Source: CAD feature listing. Evaluate the final solid. Frame: model axes, mm. A direction names the side the tool comes from. Coordinates: 2 decimals unless noted, no trailing zeros. Write each loop counter-clockwise with the first axis right and the second up, starting at its lowest first coordinate (ties: lowest second). Pieces come first, ordered by that corner, then holes. Notation, with made-up numbers: (-29, -36) -> (17, -36) arc R24 ccw to (17, -25) -> close; hole circle Ø3 at (41, 9.5). An arc over 180 degrees is marked (long way). One line per item, written item: value. Start each with the question number.
1. Section query B-B, the plane x = 214.25. Output: boundary loops of the cut face in (y, z).
2. Line query: line 1 (Y direction, x = 226.25, z = -12.25); line 2 (Y direction, x = 217.25, z = -2.25); line 3 (X direction, y = -2.25, z = -8.75). Output: solid intervals per line, ascending.
3. Section query C-C, the plane x = 227. Output: boundary loops of the cut face in (y, z), and give its area (3 significant figures).
4. First-contact query: P1, Ø4.5, axis at x = 224.5, z = -11.5, coming from the +Y side; P2, Ø4, axis at x = 214, y = -7, coming from the -Z side; P3, Ø6, axis at x = 212.5, y = -8.5, coming from the +Z side. Flat tips, straight axial feed; report the tip coordinate or a pass-through.
5. Section query D-D, the plane y = -1. Output: boundary loops of the cut face in (x, z).
6. Access query for faces 1 (the flat face through (228, -1, -9.9)), 2 (the flat face through (210.8, -11.8, -11.5)), 3 (the flat face through (228, -1, -1.2)). Directions: +Z, -Z, +X, -X, +Y, -Y. A direction counts if a zero-diameter tool reaches every point of the face in a straight line with its end or side. Return the directions, or none.
7. Section query A-A, the plane z = -13. Output: boundary loops of the cut face in (x, y).
Autodesk Inventor part; units mm, degrees
ref_plane "РабПлоскость1" through (116.75, -2.8, -7.7) normal (0, -1, 0) x (1, 0, 0)
ref_plane "YZ Plane" through (0, 0, 0) normal (1, 0, 0) x (0, 1, 0)
ref_plane "XZ Plane" through (0, 0, 0) normal (0, 1, 0) x (-1, 0, 0)
ref_plane "РабПлоскость1" through (116.75, -2.8, -7.7) normal (0, -1, 0) x (1, 0, 0)
sketch "Эскиз1" plane through (116.75, -2.8, -7.7) normal (0, -1, 0) x (1, 0, 0)
  line L0 (97, 9) -> (112.5, 9)
  line L1 (112.5, 9) -> (112.5, -9)
  line L2 (112.5, -9) -> (97, -9)
  line L3 (112.5, 2.2) -> (109.5, 2.2)
  line L4 (109.5, 2.2) -> (109.5, -6.5)
  line L5 (112.5, -6.5) -> (112.5, 2.2)
  line L6 (109.5, -6.5) -> (112.5, -6.5)
  line L7 (97, 9) -> (97, -9)
  point P0 (-116.75, 7.7)
  dimension "d9" = 15.5
  dimension "d10" = 3
  dimension "d11" = 8.7
  dimension "d13" = 2.5
extrude "Выдавливание1" add sketch "Эскиз1" along normal blind 1.5
sketch "Эскиз5" plane through (116.75, -2.8, -7.7) normal (0, 1, 0) x (1, 0, 0)
  line L0 (112.5, 9) -> (112.5, -9)
  line L1 (112.5, 2.2) -> (109.5, 2.2)
  line L2 (109.5, 2.2) -> (109.5, -6.5)
  line L3 (109.5, -6.5) -> (112.5, -6.5)
  line L4 (112.5, -6.5) -> (112.5, 2.2)
  line L5 (112.5, -9) -> (97, -9)
  point P0 (-116.75, -7.7)
  point P1 (112.5, -6.5)
  dimension "d14" = 3
  dimension "d15" = 8.7
  dimension "d16" = 2.5
extrude "Выдавливание5" add sketch "Эскиз5" along normal blind 2.8
sketch "Эскиз6" plane through (116.75, -4.3, -7.7) normal (0, -1, 0) x (1, 0, 0)
  line L0 (112.5, 9) -> (97, 9)
  line L1 (105.5, 9) -> (112.5, 9)
  line L2 (112.5, 9) -> (112.5, -9)
  line L3 (112.5, -9) -> (105.5, -9)
  line L4 (105.5, -9) -> (105.5, 9)
  point P0 (112.5, 9)
  dimension "d19" = 7
extrude "Выдавливание6" add sketch "Эскиз6" along normal blind 2.3
sketch "Эскиз7" plane through (116.75, -4.3, -7.7) normal (0, -1, 0) x (1, 0, 0)
  line L0 (97, 5.9073) -> (101.8, 5.9073)
  line L1 (101.8, 5.9073) -> (101.8, -5.6927)
  line L2 (101.8, -5.6927) -> (97, -5.6927)
  line L3 (97, -5.6927) -> (97, 5.9073)
  line L4 (97, 5.9073) -> (101.8, -5.6927) construction
  line L5 (101.8, 5.9073) -> (97, -5.6927) construction
  line L6 (97, 9) -> (97, -9)
  point P0 (99.4, 0.1073)
  point P1 (97, 0)
  dimension "d22" = 4.8
  dimension "d23" = 11.6
extrude "Выдавливание7" add sketch "Эскиз7" along normal blind 3.3
ref_plane "РабПлоскость3" through (116.75, -9.1, -7.7) normal (0, -1, 0) x (1, 0, 0)
sketch "Эскиз8" plane through (116.75, -9.1, -7.7) normal (0, -1, 0) x (1, 0, 0)
  line L0 (99.5911, -4.348) -> (90.6911, -4.348)
  line L1 (90.6911, -4.348) -> (90.6911, 4.252)
  line L2 (90.6911, 4.252) -> (99.5911, 4.252)
  line L3 (99.5911, 4.252) -> (99.5911, -4.348)
  line L4 (99.5911, -4.348) -> (90.6911, 4.252) construction
  line L5 (90.6911, -4.348) -> (99.5911, 4.252) construction
  point P0 (95.1411, -0.048)
  dimension "d27" = 8.9
  dimension "d28" = 8.6
extrude "Выдавливание8" add sketch "Эскиз8" along normal blind 2.7
sketch "Эскиз9" plane through (116.75, -11.8, -7.7) normal (0, -1, 0) x (1, 0, 0)
  line L0 (99.5911, 4.252) -> (90.6911, 4.252)
  line L1 (90.6911, 4.252) -> (90.6911, -4.348)
  line L2 (90.6911, -4.348) -> (99.5911, -4.348)
  line L3 (99.5911, -4.348) -> (99.5911, 4.252)
  circle A0 centre (95.1411, -0.048) radius 3.75
  line L4 (99.5911, -4.348) -> (99.5911, 4.252)
  line L5 (99.5911, -4.348) -> (90.6911, 4.252) construction
  line L6 (90.6911, 4.252) -> (90.6911, -4.348)
  line L7 (99.5911, 4.252) -> (90.6911, 4.252)
  line L8 (90.6911, -4.348) -> (99.5911, 4.252) construction
  point P0 (-116.75, 7.7)
  point P1 (95.1411, -0.048)
  dimension "d31" = 7.5
extrude "Выдавливание9" add sketch "Эскиз9" along normal blind 3 contours A0
sketch "Эскиз10" plane through (207.4411, -9.1, -3.448) normal (0, 0, 1) x (1, 0, 0)
  line L0 (8.9, 0) -> (8.9, -2.7)
  line L1 (8.9, -0.1624) -> (13.3567, 1.2413) construction
  line L2 (13.3567, 1.2413) -> (11.759, 4.6341) construction
  line L3 (11.759, 4.6341) -> (14.8089, 4.6341) construction
  spline S0 degree 3 poles (8.9, -0.1624) (13.3567, 1.2413) (11.759, 4.6341) (14.8089, 4.6341) knots 1 1 1 1 2 2 2 2
  line L4 (14.8089, 4.8) -> (14.8089, 2.5)
  line L5 (8.9, 0) -> (8.9, -2.7)
  line L6 (8.9, 0) -> (13.3148, 1.3302) construction
  line L7 (13.3148, 1.3302) -> (11.3789, 4.7272) construction
  line L8 (14.8089, 4.8) -> (6.3089, 4.8)
  line L9 (11.3789, 4.7272) -> (14.8089, 4.8) construction
  spline S1 degree 3 poles (8.9, 0) (13.3148, 1.3302) (11.3789, 4.7272) (14.8089, 4.8) knots 1 1 1 1 2 2 2 2
  point P0 (-207.4411, 9.1)
extrude "Выдавливание10" add sketch "Эскиз10" against normal up to surface (8.6 mm away)
properties part number "ЛЦМК0000002.00.00.00.00.04"
Computed values:
1. outline: (-14.8, -10.66) -> (-11.8, -10.66) -> (-11.8, -12.05) -> (-9.1, -12.05) -> (-9.1, -3.45) -> (-11.8, -3.45) -> (-11.8, -4.83) -> (-14.8, -4.83) -> close; (-7.6, -13.39) -> (-4.3, -13.39) -> (-4.3, -16.7) -> (-2.8, -16.7) -> (-2.8, 1.3) -> (-4.3, 1.3) -> (-4.3, -1.79) -> (-7.6, -1.79) -> close
2. line 1: y = -6.6 to -2.8
2. line 2: y = -7.6 to -2.8
2. line 3: x = 226.25 to 229.25
3. outline: (-6.6, -16.7) -> (-2.8, -16.7) -> (-2.8, -9.9) -> (0, -9.9) -> (0, -1.2) -> (-2.8, -1.2) -> (-2.8, 1.3) -> (-6.6, 1.3) -> close
3. area: 92.8 mm²
4. P1: stops at y = -2.8
4. P2: stops at z = -13.39
4. P3: stops at z = -1.79
5. outline: (226.25, -9.9) -> (229.25, -9.9) -> (229.25, -1.2) -> (226.25, -1.2) -> close
6. face 1: -Z, +X, -X, +Y
6. face 2: -Y
6. face 3: +Z, +X, -X, +Y
7. outline: (213.75, -7.6) -> (218.55, -7.6) -> (218.55, -4.3) -> (222.25, -4.3) -> (222.25, -6.6) -> (229.25, -6.6) -> (229.25, -2.8) -> (213.75, -2.8) -> close
